Model file for the job. Use its own axes, mm. A direction names the side the tool comes from. Coordinates: 2 decimals unless noted, no trailing zeros. Order: outer loops, then holes, each group sorted by start corner. A loop starts at its lowest first (then second) coordinate and runs counter-clockwise, first axis right, second up. Notation, with made-up numbers: (21, -30) - (61, -30) arc R11 cw to (61, -24) - close; hole circle Ø7 at (73.25, 41). An arc over 180 degrees is marked (long way). Put each result on its own line as item: value. Start each with the question number.
```python
from build123d import *

# Parameters (mm, degrees)
F0_W     = 31.75
F0_H     = 25.4
F0_W_2   = 19.05
F0_H_2   = 12.7
F1_DEPTH = 304.8
F2_R     = 5
F3_DEPTH = 25.4
F4_R     = 5
F5_DEPTH = 12.7


with BuildPart() as f1:
    # F0 (on Front) → F1 (new body)
    with BuildSketch(Plane.XZ):
        with Locations((1.637192, -5.449059)):
            Rectangle(F0_W, F0_H)
        with Locations((1.637192, -5.449059)):
            Rectangle(F0_W_2, F0_H_2, mode=Mode.SUBTRACT)
    extrude(amount=F1_DEPTH)

    # F2 (on face) → F3 (cut)
    with BuildSketch(Plane.YZ.offset(17.512192)):
        with Locations((-15.4, -5.449059)):
            Circle(F2_R)
        with Locations((-289.4, -5.449059)):
            Circle(F2_R)
    extrude(amount=-F3_DEPTH, mode=Mode.SUBTRACT)

    # F4 (on face) → F5 (cut)
    with BuildSketch(Plane(origin=(-14.237808, 0, 0), x_dir=(0, -1, 0), z_dir=(-1, 0, 0))):
        with Locations((144.87398, -5.449059)):
            Circle(F4_R)
        with Locations((182.974, -5.449059)):
            Circle(F4_R)
    extrude(amount=-F5_DEPTH, mode=Mode.SUBTRACT)


solid = f1.part
```
Item 1: Pull direction Y, two halves, no side cores. Call faces 4 (the face through (11.162, -150, -6)), 5 (the face through (1, -304.8, 3)), 6 (the face through (-11.107, -149.643, -3.947)), 7 (the face through (-11.107, -187.743, -3.947)): pulls with the +Y half, pulls with the -Y half, needs draft (parallel to the pull), parting line crosses it, or undercut.
Item 2: Slice it at C-C, the plane y = -15.4. Give the cut face in (x, z).
Item 3: 3-axis set-ups, long thin cutter, end or side, ignore diameter. For faces 1 (the face through (2, -150, 0.901)), 2 (the face through (14.38, -293.37, -8.49)), 3 (the face through (1, -150, -18.149)): which of +Z, -Z, +X, -X, +Y, -Y reach the whole face in a straight line?
Item 4: Flat gauge pins, fed straight in: pin 1 Ø5 at (x, z) = (-5, -7) entering from -Y; pin 2 Ø8 at (y, z) = (-15.4, -5.45) entering from +X. Where does each tip first touch, or does it go through?
Item 5: Slice it at B-B, the plane y = -199. Give the cut face in (x, z), plus the area to 3 significant figures.
Item 6: Slice it at A-A, the plane x = 3. Give the cut face in (y, z), plus the area to 3 significant figures.
Item 7: Wall check: line 1 along Z through (x, y) = (16, -15.4); line 2 along Z through (x, y) = (-1.5, -105.5); line 3 along X through (y, z) = (-230.5, -9.75). Give the ranges that are in metal, low to high.
Here are the results:
1. face 4: needs draft
1. face 5: pulls with the -Y half
1. face 6: undercut
1. face 7: undercut
2. outline: (-14.24, -18.15) - (17.51, -18.15) - (17.51, -10.45) - (11.16, -10.45) - (11.16, -11.8) - (-7.89, -11.8) - (-7.89, 0.9) - (11.16, 0.9) - (11.16, -0.45) - (17.51, -0.45) - (17.51, 7.25) - (-14.24, 7.25) - close
3. face 1: +Y, -Y
3. face 2: +X
3. face 3: -Z, +X, -X, +Y, -Y
4. pin 1: passes through
4. pin 2: stops at x = -7.89
5. outline: (-14.24, -18.15) - (17.51, -18.15) - (17.51, 7.25) - (-14.24, 7.25) - close; hole (-7.89, -11.8) - (11.16, -11.8) - (11.16, 0.9) - (-7.89, 0.9) - close
5. area: 565 mm^2
6. outline: (-304.8, -18.15) - (0, -18.15) - (0, -11.8) - (-304.8, -11.8) - close; (-304.8, 0.9) - (0, 0.9) - (0, 7.25) - (-304.8, 7.25) - close
6. area: 3,870 mm^2
7. line 1: z = -18.15 to -10.45, -0.45 to 7.25
7. line 2: z = -18.15 to -11.8, 0.9 to 7.25
7. line 3: x = -14.24 to -7.89, 11.16 to 17.51
